For this review, take the finished solid that the model builds, in its own axes (mm). Round coordinates to 2 decimals unless told otherwise and drop trailing zeros. Write each loop counter-clockwise with the first axis right and the second up, starting at its lowest first coordinate (ties: lowest second). Pieces come first, ordered by that corner, then holes.
from build123d import *

# Parameters (mm, degrees)
F0_W     = 162
F0_H     = 32
F1_DEPTH = 12
F3_D     = 8


# Not quite as in the source:
# - a pattern or mirror of a feature is missing from the dataset's text; its kind, count and spacing are read off the source's solid


with BuildPart() as f1:
    # F0 (on Front) → F1 (new body)
    with BuildSketch(Plane.XZ):
        Rectangle(F0_W, F0_H)
    extrude(amount=-F1_DEPTH)

    # F3 (through all)
    with Locations(Plane.XZ):
        with Locations((-44.5, 2)):
            f3 = Hole(F3_D / 2)

    # F3_copies: F3 across plane
    add(f3.mirror(Plane(origin=(0, 0, 0), x_dir=(0, 0, 1), z_dir=(1, 0, 0))), mode=Mode.SUBTRACT)


solid = f1.part
(1) We need section D-D, the plane x = 44. Give the boundary of the cut face in (y, z), and give its area (3 significant figures).
Geometry check:
outline: (0, -16) - (12, -16) - (12, -1.97) - (0, -1.97) - close; (0, 5.97) - (12, 5.97) - (12, 16) - (0, 16) - close
area: 289 mm2
(2) We need section C-C, the plane y = 8.5. Give the boundary of the cut face in (x, z), and give its area (3 significant figures).
Geometry check:
outline: (-81, -16) - (81, -16) - (81, 16) - (-81, 16) - close; hole circle Ø8 at (-44.5, 2); hole circle Ø8 at (44.5, 2)
area: 5,080 mm2
(3) Mouldability with a two-part tool opening along X and no side actions: class faces 1 (the face through (40.504, 6.084, 2.176)), 2 (the face through (-81, 6, 0)), 3 (the face through (-1, 6, -16)) as pulls with the +X half, pulls with the -X half, needs draft (parallel to the pull), parting line crosses it, or undercut.
Geometry check:
face 1: undercut
face 2: pulls with the -X half
face 3: needs draft
(4) For line 1 along Z through (x, y) = (44.5, 6); line 2 along X through (y, z) = (3, 0), list the stretches that pass through material, from the lowest coordinate up.
Geometry check:
line 1: z = -16 to -2, 6 to 16
line 2: x = -81 to -47.96, -41.04 to 41.04, 47.96 to 81
(5) We need section A-A, the plane x = -44.5. Give the boundary of the cut face in (y, z).
Geometry check:
outline: (0, -16) - (12, -16) - (12, -2) - (0, -2) - close; (0, 6) - (12, 6) - (12, 16) - (0, 16) - close
(6) We need section B-B, the plane z = 2. Give the boundary of the cut face in (x, y).
Geometry check:
outline: (-81, 0) - (-48.5, 0) - (-48.5, 12) - (-81, 12) - close; (-40.5, 0) - (40.5, 0) - (40.5, 12) - (-40.5, 12) - close; (48.5, 0) - (81, 0) - (81, 12) - (48.5, 12) - close
